```python
from build123d import *

# Parameters (mm, degrees)
BOSS_EXTRUDE1_DEPTH             = 4.2
SKETCH2_W                       = 4
SKETCH2_H                       = 7
BOSS_EXTRUDE2_DEPTH             = 8.6
FILLET1_R                       = 4.5
HOLE1_D                         = 3
HOLE1_DEPTH                     = 100
FILLET3_R                       = 2
FILLET4_R                       = 2
FILLET5_R                       = 3
TAP_DRILL_FOR_M2X0_4_TAP1_D     = 1.6
TAP_DRILL_FOR_M2X0_4_TAP1_DEPTH = 1.98
TAP_DRILL_FOR_M2X0_4_TAP1_TIP   = 0.480688495


with BuildPart() as part:
    # Sketch1 → Boss-Extrude1 (new body)
    with BuildSketch(Plane.XY):
        with BuildLine():
            Line((4, 26), (4, 24.096998671))
            ThreePointArc((4, 24.096998671), (6.041195573, 23.890909602), (8, 23.280961007))
            Line((8, 23.280961007), (8, 26))
            Line((8, 26), (4, 26))
        make_face()
        with BuildLine():
            ThreePointArc((8, 23.280961007), (6.041195573, 23.890909602), (4, 24.096998671))
            Line((4, 24.096998671), (4, 21.096998671))
            ThreePointArc((4, 21.096998671), (6.089651945, 20.787605561), (8, 19.885973898))
            Line((8, 19.885973898), (8, 23.280961007))
        make_face()
        with BuildLine():
            ThreePointArc((8, 19.885973898), (6.089651945, 20.787605561), (4, 21.096998671))
            Line((4, 21.096998671), (4, 19))
            Line((4, 19), (8, 19))
            Line((8, 19), (8, 19.885973898))
        make_face()
        with BuildLine():
            Line((4, 21.096998671), (4, 24.096998671))
            ThreePointArc((4, 24.096998671), (1.958804427, 23.890909602), (0, 23.280961007))
            Line((0, 23.280961007), (0, 19.885973898))
            ThreePointArc((0, 19.885973898), (1.910348055, 20.787605561), (4, 21.096998671))
        make_face()
        with BuildLine():
            Line((0, 7.885047636), (0, 4.490060527))
            ThreePointArc((0, 4.490060527), (1.958804427, 3.880111932), (4, 3.674022863))
            Line((4, 3.674022863), (4, 6.674022863))
            ThreePointArc((4, 6.674022863), (1.910348055, 6.983415973), (0, 7.885047636))
        make_face()
        with BuildLine():
            Line((0, 19.885973898), (0, 23.280961007))
            ThreePointArc((0, 23.280961007), (-6.211487904, 13.885510767), (0, 4.490060527))
            Line((0, 4.490060527), (0, 7.885047636))
            ThreePointArc((0, 7.885047636), (-3.211487904, 13.885510767), (0, 19.885973898))
        make_face()
        with BuildLine():
            ThreePointArc((4, 3.674022863), (1.958804427, 3.880111932), (0, 4.490060527))
            Line((0, 4.490060527), (0, 0))
            Line((0, 0), (8, 0))
            Line((8, 0), (8, 4.490060527))
            ThreePointArc((8, 4.490060527), (6.041195573, 3.880111932), (4, 3.674022863))
        make_face()
        with BuildLine():
            Line((8, 10), (4, 10))
            Line((4, 10), (4, 6.674022863))
            ThreePointArc((4, 6.674022863), (6.089651945, 6.983415973), (8, 7.885047636))
            Line((8, 7.885047636), (8, 10))
        make_face()
        with BuildLine():
            Line((4, 6.674022863), (4, 10))
            Line((4, 10), (0, 10))
            Line((0, 10), (0, 7.885047636))
            ThreePointArc((0, 7.885047636), (1.910348055, 6.983415973), (4, 6.674022863))
        make_face()
        with BuildLine():
            ThreePointArc((4, 3.674022863), (6.041195573, 3.880111932), (8, 4.490060527))
            Line((8, 4.490060527), (8, 7.885047636))
            ThreePointArc((8, 7.885047636), (6.089651945, 6.983415973), (4, 6.674022863))
            Line((4, 6.674022863), (4, 3.674022863))
        make_face()
    extrude(amount=BOSS_EXTRUDE1_DEPTH)

    # Sketch2 → Boss-Extrude2 (add)
    with BuildSketch(Plane.XY.offset(4.2)):
        with Locations((6, 22.5)):
            Rectangle(SKETCH2_W, SKETCH2_H)
    extrude(amount=BOSS_EXTRUDE2_DEPTH)

    # Fillet1
    fillet1_edges = [part.edges().sort_by_distance(p)[0] for p in [
        (8, 0, 2.1),
    ]]
    fillet(fillet1_edges, radius=FILLET1_R)

    # Hole1
    with Locations(Plane(origin=(3.5, 4.6, 4.2), x_dir=(1, 0, 0), z_dir=(0, 0, 1))):
        with Locations((0, 0)):
            Hole(HOLE1_D / 2, depth=HOLE1_DEPTH)

    # Fillet3
    fillet3_edges = [part.edges().sort_by_distance(p)[0] for p in [
        (0, 10, 2.1),
    ]]
    fillet(fillet3_edges, radius=FILLET3_R)

    # Fillet4
    fillet4_edges = [part.edges().sort_by_distance(p)[0] for p in [
        (8, 19, 6.4),
        (4, 19, 6.4),
    ]]
    fillet(fillet4_edges, radius=FILLET4_R - 0.0001)  # a hair under: the kernel refuses the full size

    # Fillet5
    fillet5_edges = [part.edges().sort_by_distance(p)[0] for p in [
        (0, 0, 2.1),
    ]]
    fillet(fillet5_edges, radius=FILLET5_R)

    # Tap Drill for M2x0.4 Tap1
    with Locations(Plane(origin=(8, 7.5, 2.1), x_dir=(0, 0, 1), z_dir=(1, 0, 0))):
        with Locations((0, 0)):
            Hole(TAP_DRILL_FOR_M2X0_4_TAP1_D / 2, depth=TAP_DRILL_FOR_M2X0_4_TAP1_DEPTH)
            with Locations((0, 0, -(TAP_DRILL_FOR_M2X0_4_TAP1_DEPTH + TAP_DRILL_FOR_M2X0_4_TAP1_TIP / 2))):  # 118° drill point
                Cone(0, TAP_DRILL_FOR_M2X0_4_TAP1_D / 2, TAP_DRILL_FOR_M2X0_4_TAP1_TIP, mode=Mode.SUBTRACT)


solid = part.part
```
Check sheet for the modelled part. Datum: model origin and axes. Units: mm. A direction names the side the tool comes from. Coordinates: 2 decimals unless noted, no trailing zeros. Order: outer loops, then holes, each group sorted by start corner. A loop starts at its lowest first (then second) coordinate and runs counter-clockwise, first axis right, second up. Notation, with made-up numbers: (-38.5, 26) -> (5.5, 26) arc R6 ccw to (5.5, 37) -> close; hole circle Ø5 at (-19, -8). An arc over 180 degrees is marked (long way). Write each question's results on one line, items separated by ' | '. Start each with the question number.
1) Draft check along X on faces 1 (the face through (4.57, 19.6, 6.49)), 2 (the face through (-4, 13, 0)), 3 (the face through (8, 23, 6)). Enter one of: pulls with the +X half, pulls with the -X half, needs draft (parallel to the pull), parting line crosses it, or undercut.
2) Depth check by flat-ended pin: pin 1 (1.5 mm diameter, centred on x = 0, y = 16.5, fed in from +Z); pin 2 (2 mm diameter, centred on x = -4.5, z = 2, fed in from -Y); pin 3 (2.5 mm diameter, centred on y = 22.5, z = 6.5, fed in from -X); pin 4 (4 mm diameter, centred on x = 6.5, y = 9, fed in from +Z). Enter the tip coordinate at first touch or a pass-through.
3) Set-up check for faces 4 (the face through (0.6, 9.43, 2.13)), 5 (the face through (7.4, 19.57, 6.49)), 6 (the face through (6.996, 7.26, 1.337)): record each of +Z, -Z, +X, -X, +Y, -Y from which the full face is reachable in a straight line by a thin tool's end or side.
4) Section check A-A (y = 9.5). Enter the section's corners in (x, z), and give its area (3 significant figures).
5) Section check B-B (x = 4.5). Enter the section's corners in (y, z).
6) Material ranges on line 1 along Z through (x, y) = (7.15, 7.5); line 2 along X through (y, z) = (25.25, 7.75); line 3 along Z through (x, y) = (-2.5, 20), recorded low to high.
7) Section check D-D (y = 24.75). Enter the section's corners in (x, z), and give its area (3 significant figures).
Checked values:
1) face 1: undercut | face 2: needs draft | face 3: pulls with the +X half
2) pin 1: through | pin 2: y = 6.96 | pin 3: x = 4 | pin 4: z = 4.2
3) face 4: +Z, -Z | face 5: +Z, -Z, +X | face 6: +X
4) outline: (-5.22, 0) -> (-1.72, 0) -> (-1.72, 4.2) -> (-5.22, 4.2) -> close; (0.68, 0) -> (8, 0) -> (8, 4.2) -> (0.68, 4.2) -> close | area: 45.4 mm²
5) outline: (0.11, 0) -> (3.48, 0) -> (3.48, 4.2) -> (0.11, 4.2) -> close; (5.72, 0) -> (10, 0) -> (10, 4.2) -> (5.72, 4.2) -> close; (19.68, 0) -> (26, 0) -> (26, 12.8) -> (19.68, 12.8) -> close
6) line 1: 0 to 1.3, 2.9 to 4.2 | line 2: 4 to 8 | line 3: 0 to 4.2
7) outline: (4, 0) -> (8, 0) -> (8, 12.8) -> (4, 12.8) -> close | area: 51.2 mm²
